Geometry check sheet. Reference: drawing and pictorial views, mm from the part's lowest x, y, z. Give positions to 0.01 mm unless a question says otherwise; leave off trailing zeros. Loops run counter-clockwise (first coordinate to the right, second up) from the corner with the lowest first, then second, coordinate; pieces in that order, holes last. Notation, with made-up numbers: (-17.5, 52.25) - (9.5, 52.25) arc R16 cw to (9.5, 76.25) - close; hole circle Ø4 at (66, 15). An arc over 180 degrees is marked (long way). One line per question, with ' | ' between items. Start each with the question number.
1. Section check A-A, the plane y = 54. Enter the section's corners in (x, z).
2. Section check C-C, the plane x = 69. Enter the section's corners in (y, z), then the cut area to 3 significant figures.
3. Section check B-B, the plane z = 3.25. Enter the section's corners in (x, y).
4. Thickness scan on line 1 along X through (y, z) = (58.5, 0.55); line 2 along X through (y, z) = (63, 2.35); line 3 along Y through (x, z) = (38.5, 2.2). Record the ranges inside material, lowest first. Write a range as from..to.
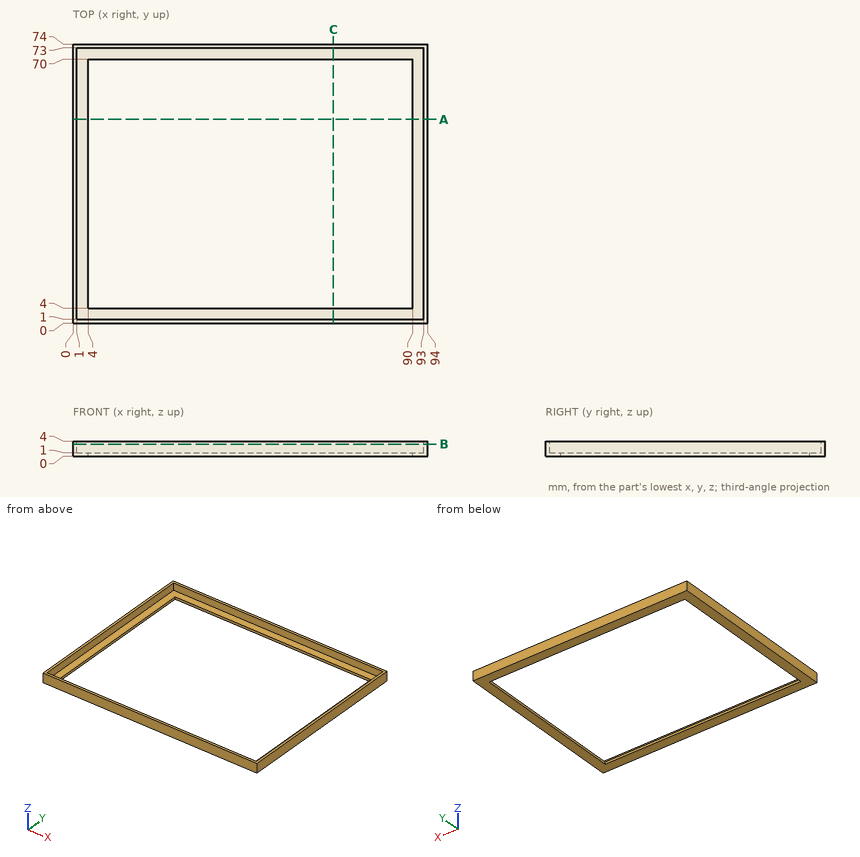
Results list:
1) outline: (0, 0) - (4, 0) - (4, 1) - (1, 1) - (1, 4) - (0, 4) - close; (90, 0) - (94, 0) - (94, 4) - (93, 4) - (93, 1) - (90, 1) - close
2) outline: (0, 0) - (4, 0) - (4, 1) - (1, 1) - (1, 4) - (0, 4) - close; (70, 0) - (74, 0) - (74, 4) - (73, 4) - (73, 1) - (70, 1) - close | area: 14.0 mm²
3) outline: (0, 0) - (94, 0) - (94, 74) - (0, 74) - close; hole (1, 1) - (93, 1) - (93, 73) - (1, 73) - close
4) line 1: 0..4, 90..94 | line 2: 0..1, 93..94 | line 3: 0..1, 73..74
